Read the model definition and answer for the solid it produces. Units are mm, in the model's axes. Give positions to 0.01 mm unless a question says otherwise; leave off trailing zeros. Order: outer loops, then holes, each group sorted by start corner. A loop starts at its lowest first (then second) coordinate and runs counter-clockwise, first axis right, second up. Notation, with made-up numbers: M -24,53.5 L 6,53.5 A25 cw 6,76.5 Z; hole C -23,86 d2. An arc over 180 degrees is marked long. One line per item, written item: value.
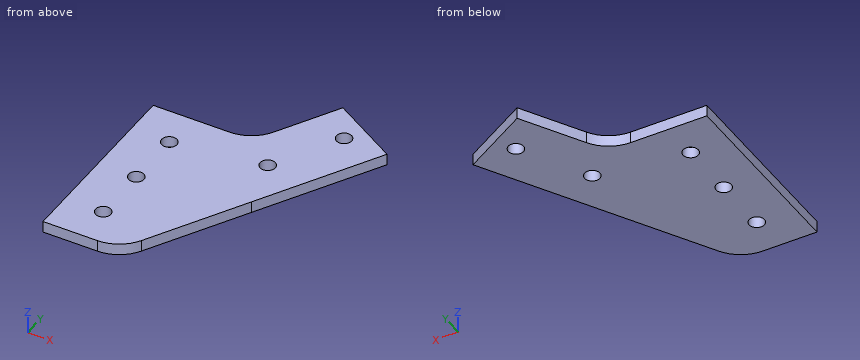
from build123d import *

# Parameters (mm, degrees)
SKETCH_1_R      = 2
SKETCH_1_W      = 20
SKETCH_1_H      = 50
EXTRUDE_1_DEPTH = 3
FILLET_1_R      = 10


with BuildPart() as part:
    # 草图1 → 凸台-拉伸1 (new body)
    # profile 1 of 3: a face of its own
    with BuildSketch(Plane.XY):
        Polygon((27.320508076, 5), (10, 15), (10, -25), align=None)
    # profile 2 of 3: a face of its own
    with BuildSketch(Plane.XY):
        Polygon((27.735682985, 45.719104037), (45.05619106, 35.719104037), (27.320508076, 5), (10, 15), align=None)
        with Locations((33.660254038, 35.980762114)):
            Circle(SKETCH_1_R, mode=Mode.SUBTRACT)
        with Locations((23.660254038, 18.660254038)):
            Circle(SKETCH_1_R, mode=Mode.SUBTRACT)
    # profile 3 of 3: a face of its own
    with BuildSketch(Plane.XY):
        Rectangle(SKETCH_1_W, SKETCH_1_H)
        Circle(SKETCH_1_R, mode=Mode.SUBTRACT)
        with Locations((0, -15)):
            Circle(SKETCH_1_R, mode=Mode.SUBTRACT)
        with Locations((0, 15)):
            Circle(SKETCH_1_R, mode=Mode.SUBTRACT)
    extrude(amount=EXTRUDE_1_DEPTH)

    # 圆角1
    # the kernel refuses this fillet: 10 mm, written as the material it adds along each edge
    with BuildSketch(Plane(origin=(10, 15, 0), x_dir=(0.49999999999999756, 0.86602540378444, 0), z_dir=(0, 0, 1))) as fillet_1_piece_1:
        with BuildLine():
            CenterArc((17.320508076, 10), FILLET_1_R, 210, 60)
            Line((8.660254038, 5), (0, 0))
            Line((0, 0), (17.320508076, 0))
        make_face()
    extrude(amount=3)
    # the kernel refuses this fillet: 10 mm, written as the material it takes off along each edge
    with BuildSketch(Plane(origin=(10, -25, -14.43375673), x_dir=(0.49999999999999745, 0.86602540378444, 0), z_dir=(0, 0, 1))) as fillet_1_2_piece_1:
        with BuildLine():
            CenterArc((FILLET_1_R * 0.57735026919, FILLET_1_R), FILLET_1_R, 210, 60)
            Line((-FILLET_1_R * 0.288675134595, FILLET_1_R * 0.5), (0, 0))
            Line((0, 0), (FILLET_1_R * 0.57735026919, 0))
        make_face()
    extrude(amount=31.867513459, mode=Mode.SUBTRACT)


solid = part.part
1) Consider probe 1 along Y at (x, z) = (0, 1.25); probe 2 along Y at (x, z) = (3, 0.7); probe 3 along X at (y, z) = (-20, 0.5). Determine where each line is inside the solid, lowest interval first.
Reported:
probe 1: y = -25 to -17, -13 to -2, 2 to 13, 17 to 25
probe 2: y = -25 to 25
probe 3: x = -10 to 12.89
2) Find section C-C, the plane z = 2.3. Write down the section's boundary in (x, y).
Reported:
outline: M -10,-25 L 4.23,-25 A10 ccw 12.89,-20 L 45.06,35.72 L 27.74,45.72 L 18.66,30 A10 cw 10,25 L -10,25 Z; hole C 0,-15 d4; hole C 0,0 d4; hole C 0,15 d4; hole C 23.66,18.66 d4; hole C 33.66,35.98 d4
3) Find section A-A, the plane x = 0. Write down the section's boundary in (y, z).
Reported:
outline: M -25,0 L -17,0 L -17,3 L -25,3 Z; M -13,0 L -2,0 L -2,3 L -13,3 Z; M 2,0 L 13,0 L 13,3 L 2,3 Z; M 17,0 L 25,0 L 25,3 L 17,3 Z
4) Find section D-D, the plane x = 34.5. Write down the section's boundary in (y, z), plus the area to 3 significant figures.
Reported:
outline: M 17.44,0 L 34.17,0 L 34.17,3 L 17.44,3 Z; M 37.8,0 L 41.81,0 L 41.81,3 L 37.8,3 Z
area: 62.2 mm^2
5) Find section B-B, the plane y = 15. Write down the section's boundary in (x, z).
Reported:
outline: M -10,0 L -2,0 L -2,3 L -10,3 Z; M 2,0 L 33.09,0 L 33.09,3 L 2,3 Z
